Geometry: final body of the model. Coordinates: model frame, mm. Face numbers are marked on the shaded views. A direction names the side the tool comes from. Give positions to 0.01 mm unless a question says otherwise; leave off trailing zeros. Write each loop counter-clockwise with the first axis right and the second up, starting at its lowest first coordinate (ties: lowest second). Pieces come first, ordered by that corner, then holes.
Q1. Cut plane B-B on z = 12. Return the cut outline in (x, y) (3 decimals).
Q2. Cut plane D-D on y = 4.5. Return the cut outline in (x, z) (3 decimals).
Q3. Cut plane C-C on x = 1. Return the cut outline in (y, z), plus the area to 3 significant figures.
Q4. Line query: L1, parallel to X at y = 17, z = 10.75 (3 decimals); L2, parallel to Y at x = -4.5, z = 8.5; L3, parallel to Y at x = -7.5, z = 12. Output: solid intervals per line, ascending.
Q5. Cut plane A-A on y = 20. Return the cut outline in (x, z) (3 decimals), plus the area to 3 significant figures.
Q6. Pin query (flat end, axial travel): pin 1 (3 mm diameter, centred on x = 12, y = 4, fed in from +Z) (3 decimals); pin 2 (4.5 mm diameter, centred on x = -3, z = 14, fed in from -Y). Return the tip coordinate at first contact, or that it passes through.
Q7. Reachability of the marked faces 4 and 5 from +Z, -Z, +X, -X, +Y, -Y: full face, straight path, thin tool, end or side. Return the list, or none.
Q8. Draft query along X for the marked faces 1, 2 and 3. Return one class per face: pulls with the +X half, pulls with the -X half, needs draft (parallel to the pull), parting line crosses it, or undercut.
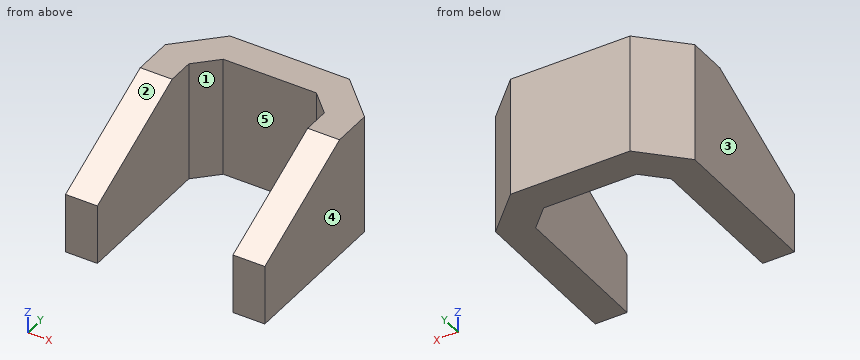
```python
from build123d import *

# Parameters (mm, degrees)
F1_DEPTH = 19.05
F2_T     = -5.08
F4_DEPTH = 31.751


with BuildPart() as f1:
    # F0 (on Top) → F1 (new body)
    with BuildSketch(Plane.XY):
        Polygon((-15.875, 25.4), (-15.875, 0), (15.875, 0), (15.875, 25.4), (9.525, 31.75), (-9.525, 31.75), align=None)
    extrude(amount=F1_DEPTH)

    # F2
    f2_openings = [f1.faces().sort_by_distance(p)[0] for p in [
        (0, 15.301736, 19.05),
        (0, 0, 9.525),
        (0, 15.301736, 0),
    ]]
    offset(amount=F2_T, openings=f2_openings)

    # F3 (on face) → F4 (cut, through all)
    with BuildSketch(Plane.YZ.offset(15.875)):
        Polygon((0, 19.05), (0, 9.525), (19.05, 19.05), align=None)
    extrude(amount=-F4_DEPTH, mode=Mode.SUBTRACT)


solid = f1.part
```
Data:
1. outline: (-15.875, 4.95) - (-10.795, 4.95) - (-10.795, 23.296) - (-7.421, 26.67) - (7.421, 26.67) - (10.795, 23.296) - (10.795, 4.95) - (15.875, 4.95) - (15.875, 25.4) - (9.525, 31.75) - (-9.525, 31.75) - (-15.875, 25.4) - close
2. outline: (-15.875, 0) - (-10.795, 0) - (-10.795, 11.775) - (-15.875, 11.775) - close; (10.795, 0) - (15.875, 0) - (15.875, 11.775) - (10.795, 11.775) - close
3. outline: (26.67, 0) - (31.75, 0) - (31.75, 19.05) - (26.67, 19.05) - close
3. area: 96.8 mm2
4. L1: x = -15.875 to -10.795, 10.795 to 15.875
4. L2: y = 26.67 to 31.75
4. L3: y = 26.59 to 31.75
5. outline: (-15.875, 0) - (-10.795, 0) - (-10.795, 19.05) - (-15.875, 19.05) - close; (10.795, 0) - (15.875, 0) - (15.875, 19.05) - (10.795, 19.05) - close
5. area: 194 mm2
6. pin 1: stops at z = 12.275
6. pin 2: stops at y = 26.67
7. face 4: +Z, -Z, +X, +Y, -Y
7. face 5: +Z, -Z, -Y
8. face 1: undercut
8. face 2: needs draft
8. face 3: pulls with the -X half
